The listing builds one solid part. Answer for the finished solid, in the listing's coordinates (mm). A direction names the side the tool comes from. Give positions to 0.01 mm unless a question says otherwise; leave off trailing zeros. Write each loop counter-clockwise with the first axis right and the second up, starting at its lowest first coordinate (ties: lowest second). Pieces come first, ordered by that corner, then holes. Notation, with made-up numbers: M 80.5,2.25 L 95.5,2.25 A20 ccw 95.5,28.25 Z; hole C -24,54.5 d11. An arc over 180 degrees is marked long. Return JSON: item names as keys, results as strings.
from build123d import *

# Parameters (mm, degrees)
FILLET2_R = 2


with BuildPart() as part:
    # Sketch1 → Revolve1 (revolve)
    with BuildSketch(Plane.XY, mode=Mode.PRIVATE) as revolve1_sk:
        Polygon((10, -20), (12, -20), (14.459464607, -2.5), (36, -2.5), (36, -14.5), (40, -14.5), (40, 14.5), (36, 14.5), (36, 2.5), (14.459464607, 2.5), (12, 20), (10, 20), align=None)
    revolve(revolve1_sk.sketch.rotate(Axis((0, -24.578986378, 0), (0, 1, 0)), 90), axis=Axis((0, -24.578986378, 0), (0, 1, 0)))

    # Fillet2
    fillet2_edges = [part.edges().sort_by_distance(p)[0] for p in [
        (0, 14.5, 36),
        (0, 14.5, 40),
        (0, -14.5, 40),
        (0, -14.5, 36),
    ]]
    fillet(fillet2_edges, radius=FILLET2_R - 0.0001)  # a hair under: the kernel refuses the full size


solid = part.part
Item 1: Given pin 1 Ø3 at (x, y) = (7, -6.5) entering from -Z; pin 2 Ø1.5 at (y, z) = (1, -15) entering from +X; pin 3 Ø4 at (y, z) = (-11.5, 26) entering from +X, each flat-ended and moving along its own axis, determine where each tip first touches the part or whether it passes through.
Geometry results:
{"pin 1": "stops at z = -39.62", "pin 2": "stops at x = 37.38", "pin 3": "stops at x = 32"}
Item 2: Which of the six approach directions +Z, -Z, +X, -X, +Y, -Y give full straight-line access (tool end or side, diameter ignored) to faces 1 (the flat face through (-9, -20, -5)), 2 (the cylindrical face through (-24.331, 7.43, 26.533)), 3 (the flat face through (15, -2.5, -1))?
Geometry results:
{"face 1": "+Z, -Z, +X, -X, -Y", "face 2": "+Y", "face 3": "-Y"}
Item 3: Determine the mould class of faces 4 (the flat face through (-9, 20, 5)), 5 (the cylindrical face through (-1.76, 0.18, 39.96)), 6 (the cylindrical face through (0, 0, 10)) for opening direction X: +X half, -X half, draft (parallel to the pull), parting line (faces both ways), or undercut.
Geometry results:
{"face 4": "draft", "face 5": "parting line", "face 6": "undercut"}
Item 4: A cutting plane is placed at C-C, the plane y = 11.5. Write down the section's boundary in (x, z), plus the area to 3 significant figures.
Geometry results:
{"outline": "C 0,0 d80; C 0,0 d26.39; hole C 0,0 d72; hole C 0,0 d20", "area": "1,190 mm2"}
Item 5: A cutting plane is placed at D-D, the plane y = -7. Write down the section's boundary in (x, z), plus the area to 3 significant figures.
Geometry results:
{"outline": "C 0,0 d80; C 0,0 d27.65; hole C 0,0 d72; hole C 0,0 d20", "area": "1,240 mm2"}
Item 6: Find the intervals of material crossed by line 1 (Z direction, x = -2, y = -8); line 2 (X direction, y = -9, z = 0); line 3 (X direction, y = 6, z = 0), in increasing order.
Geometry results:
{"line 1": "z = -39.95 to -35.94, -13.54 to -9.8, 9.8 to 13.54, 35.94 to 39.95", "line 2": "x = -40 to -36, -13.55 to -10, 10 to 13.55, 36 to 40", "line 3": "x = -40 to -36, -13.97 to -10, 10 to 13.97, 36 to 40"}
